Autodesk Inventor part; units mm, degrees
ref_plane "YZ Plane" through (0, 0, 0) normal (1, 0, 0) x (0, 1, 0)
ref_plane "XZ Plane" through (0, 0, 0) normal (0, 1, 0) x (-1, 0, 0)
ref_plane "XY Plane" through (0, 0, 0) normal (0, 0, 1) x (1, 0, 0)
sketch "Esboço1" plane through (0, 0, 0) normal (0, 0, 1) x (1, 0, 0)
  line L0 (136.913, 75.5114) -> (56.913, 75.5114)
  line L1 (56.913, 75.5114) -> (42.913, 114.5391)
  line L2 (42.913, 114.5391) -> (-117.087, 114.5391)
  line L3 (-117.087, 114.5391) -> (-117.087, -114.7608)
  line L4 (136.913, 75.5114) -> (136.913, -89.3608)
  line L5 (136.913, -89.3608) -> (-117.087, -114.7608)
  line L6 (136.913, 46.0024) -> (136.913, 42.8274)
  line L7 (-116.1736, -114.6695) -> (137.8264, -89.2695)
  circle A0 centre (85.351, 57.8134) radius 3.3782
  circle A1 centre (-42.3105, 57.8134) radius 4.7625
  circle A2 centre (-42.3105, 83.2134) radius 4.7625
  circle A3 centre (-56.9241, 100.9934) radius 4.7625
  circle A4 centre (-24.4105, 100.9934) radius 4.7625
  circle A5 centre (-42.3105, 108.6134) radius 4.7625
  circle A6 centre (-67.049, 57.8134) radius 3.3782
  circle A7 centre (-1.5943, 83.2134) radius 11.1125
  circle A8 centre (-16.249, 57.8134) radius 3.3782
  circle A9 centre (3.0987, 100.9934) radius 4.7625
  circle A10 centre (-16.249, 108.6134) radius 3.3782
  circle A11 centre (-67.049, 108.6134) radius 3.3782
  circle A12 centre (-117.849, 57.8134) radius 6.096
  line L8 (129.1695, -83.1003) -> (-109.6394, -106.9812)
  arc A13 (129.1695, -83.1003) -> (128.5725, -77.1301) centre (128.871, -80.1152) ccw
  line L9 (-110.2364, -101.011) -> (128.5725, -77.1301)
  arc A14 (-110.2364, -101.011) -> (-109.6394, -106.9812) centre (-109.9379, -103.9961) ccw
  line L10 (-97.087, 114.5391) -> (-117.087, 114.5391)
  line L11 (-117.087, 114.5391) -> (-117.087, 35.1191)
  line L12 (-117.087, 35.1191) -> (-97.087, 35.1191)
  line L13 (-97.087, 35.1191) -> (-97.087, 114.5391)
  point P0 (0, 0)
  point P1 (-117.087, 63.8616)
  point P2 (-117.087, 51.7652)
  dimension "d0" = 254
  dimension "d1" = 80
  dimension "d2" = 160
  dimension "d3" = 109.734
  dimension "d6" = 20
extrude "Extrusão1" add sketch "Esboço1" along normal blind 5 contours L4 L5 L3 L12 L13 L2 L1 L0
fillet "Arredondamento1" radius 10 6 edges at (-97.087, 35.1191, 2.5) (-117.087, 35.1191, 2.5) (-97.087, 114.5391, 2.5) (42.913, 114.5391, 2.5) (56.913, 75.5114, 2.5) (136.913, 75.5114, 2.5)
properties part number "CHAPA FIXAÇÃO DIREITA 1"
Geometry: final body of the model. Coordinates: model frame, mm. A direction names the side the tool comes from. Coordinates: 2 decimals unless noted, no trailing zeros. Write each loop counter-clockwise with the first axis right and the second up, starting at its lowest first coordinate (ties: lowest second). Pieces come first, ordered by that corner, then holes. Notation, with made-up numbers: M 81,22 L 121,22 A26 cw 121,40 Z; hole C -2,70.5 d3. An arc over 180 degrees is marked long. Use CSV: the item, a comma, the result in double quotes. Start each with the question number.
1. Cut plane C-C on z = 2. Count the separate pieces of the cut face and the enclosed holes in it, plus the area to 3 significant figures.
2. Mould query, pull axis X, two halves, no side actions, for faces 3 (the face through (-100.094, 37.971, 2.535)), 4 (the face through (58.1, 77.4, 2.5)), 5 (the face through (4.38, 73.843, 2.465)). Classes: pulls with the +X half, pulls with the -X half, needs draft (parallel to the pull), parting line crosses it, or undercut.
3. Cut plane A-A on x = 92. Return the cut outline in (y, z).
4. Cut plane D-D on x = 12.5. Return the cut outline in (y, z).
5. Cut plane B-B on x = -41. Return the cut outline in (y, z), plus the area to 3 significant figures.
6. Ray query, probe 1 along Y at (x, z) = (-64, 3.35); probe 2 along Y at (x, z) = (-42, 1.35); probe 3 along X at (y, z) = (50, 2.1). Return the intervals inside material, ascending.
7. First-contact query: P1, Ø7.5, axis at x = -42.31, y = 108.61, coming from the -Z side. Flat tip, straight axial feed; report the tip coordinate or a pass-through.
8. Reachability of faces 1 (the face through (134.062, 72.504, 2.535)), 2 (the face through (7.496, -89.238, 2.465)) from +Z, -Z, +X, -X, +Y, -Y: full face, straight path, thin tool, end or side. Return the list, or none.
Entries:
1,separate pieces,"1"
1,enclosed holes,"13"
1,area,"47,500 mm²"
2,face 3,"pulls with the -X half"
2,face 4,"pulls with the +X half"
2,face 5,"undercut"
3,outline,"M -93.85,0 L -86.82,0 L -86.82,5 L -93.85,5 Z; M -80.79,0 L 75.51,0 L 75.51,5 L -80.79,5 Z"
4,outline,"M -101.8,0 L -94.77,0 L -94.77,5 L -101.8,5 Z; M -88.74,0 L 114.54,0 L 114.54,5 L -88.74,5 Z"
5,outline,"M -107.15,0 L -100.12,0 L -100.12,5 L -107.15,5 Z; M -94.09,0 L 53.23,0 L 53.23,5 L -94.09,5 Z; M 62.39,0 L 78.63,0 L 78.63,5 L 62.39,5 Z; M 87.79,0 L 104.03,0 L 104.03,5 L 87.79,5 Z; M 113.19,0 L 114.54,0 L 114.54,5 L 113.19,5 Z"
5,area,"941 mm²"
6,probe 1,"-109.45 to -102.42, -96.39 to 56.36, 59.27 to 107.16, 110.07 to 114.54"
6,probe 2,"-107.25 to -100.22, -94.19 to 53.06, 62.57 to 78.46, 87.97 to 103.86, 113.37 to 114.54"
6,probe 3,"-97.09 to 136.91"
7,P1,"through"
8,face 1,"+Z, -Z, +X, +Y"
8,face 2,"+Z, -Z"
